Geometry check sheet. Reference: the model listing, model coordinates, mm. A direction names the side the tool comes from. Give positions to 0.01 mm unless a question says otherwise; leave off trailing zeros. Order: outer loops, then holes, each group sorted by start corner. A loop starts at its lowest first (then second) coordinate and runs counter-clockwise, first axis right, second up. Notation, with made-up numbers: M 33,59 L 58,59 A30 cw 58,83 Z; hole C -28.5,-15 d9. An arc over 180 degrees is marked long. One line per question, with ' | ' between items. Start each with the question number.
Autodesk Inventor part; units mm, degrees
ref_plane "YZ Plane" through (0, 0, 0) normal (1, 0, 0) x (0, 1, 0)
ref_plane "XZ Plane" through (0, 0, 0) normal (0, 1, 0) x (-1, 0, 0)
ref_plane "XY Plane" through (0, 0, 0) normal (0, 0, 1) x (1, 0, 0)
sketch "Sketch1" plane through (0, 0, 0) normal (0, 1, 0) x (-1, 0, 0)
  line L0 (0, 0) -> (0, -25.4)
  line L1 (0, -25.4) -> (3.175, -25.4)
  line L2 (3.175, -25.4) -> (3.175, -3.175)
  line L3 (3.175, -3.175) -> (25.4, -3.175)
  line L4 (25.4, -3.175) -> (25.4, 0)
  line L5 (25.4, 0) -> (0, 0)
  dimension "d0" = 3.175
  dimension "d1" = 3.175
  dimension "d2" = 25.4
  dimension "d3" = 25.4
extrude "Extrusion1" add sketch "Sketch1" along normal blind 177.8
sketch "Sketch2" plane through (-25.4, 0, 0) normal (0, 0, 1) x (1, 0, 0)
  line L0 (0, 177.8) -> (25.4, 177.8)
  line L1 (0, 0) -> (25.4, 0)
  line L2 (0, 0) -> (0, 177.8)
  point P0 (12.7, 165.1)
  point P1 (12.7, 12.7)
  dimension "d6" = 12.7
  dimension "d7" = 12.7
  dimension "d8" = 12.7
  dimension "d9" = 12.7
hole "Hole1" at (-12.7, 165.1, 0) at (-12.7, 12.7, 0) direction (0, 0, -1) diameter 6.7469 end through all
properties part number "15102898-16-P-0312"
Item 1: Cross-section at A-A, the plane x = -12.7. Record the cut outline in (y, z) (3 decimals), plus the area to 3 significant figures.
Item 2: Cross-section at D-D, the plane z = -9.5. Record the cut outline in (x, y) (3 decimals), plus the area to 3 significant figures.
Item 3: Depth check by flat-ended pin: pin 1 (11 mm diameter, centred on x = -11, y = 80.5, fed in from -Z) (3 decimals); pin 2 (5.5 mm diameter, centred on x = -12.7, y = 165.1, fed in from +Z). Enter the tip coordinate at first touch or a pass-through.
Item 4: Material ranges on line 1 along Y through (x, z) = (-12.7, -1.45); line 2 along X through (y, z) = (165.1, -2.1); line 3 along X through (y, z) = (132, -10) (3 decimals), recorded low to high.
Item 5: Set-up check for faces 1 (the flat face through (-14, 88, -3.175)), 2 (the flat face through (0, 88, -13)): record each of +Z, -Z, +X, -X, +Y, -Y from which the full face is reachable in a straight line by a thin tool's end or side.
Item 6: Cross-section at B-B, the plane y = 165.1. Record the cut outline in (x, z) (3 decimals).
Item 7: Mould release check, pull along Y, two halves, no side actions. Record for faces 3 (the flat face through (-2, 177.8, -7)), 4 (the flat face through (-25.4, 88, -2)), 5 (the cylindrical face through (-12.85, 168.47, -1.61)), 6 (the flat face through (-2, 0, -7)): released by +Y, released by -Y, zero draft, split by the parting line, or undercut.
Item 8: Cross-section at C-C, the plane y = 65. Record the cut outline in (x, z) (3 decimals).
Outcome:
1) outline: M 0,-3.175 L 9.327,-3.175 L 9.327,0 L 0,0 Z; M 16.073,-3.175 L 161.727,-3.175 L 161.727,0 L 16.073,0 Z; M 168.473,-3.175 L 177.8,-3.175 L 177.8,0 L 168.473,0 Z | area: 522 mm²
2) outline: M -3.175,0 L 0,0 L 0,177.8 L -3.175,177.8 Z | area: 565 mm²
3) pin 1: stops at z = -3.175 | pin 2: passes through
4) line 1: y = 0 to 9.33, 16.07 to 161.73, 168.47 to 177.8 | line 2: x = -25.4 to -16.07, -9.33 to 0 | line 3: x = -3.175 to 0
5) face 1: -Z, -X, +Y, -Y | face 2: +Z, -Z, +X, +Y, -Y
6) outline: M -25.4,-3.175 L -16.073,-3.175 L -16.073,0 L -25.4,0 Z; M -9.327,-3.175 L -3.175,-3.175 L -3.175,-25.4 L 0,-25.4 L 0,0 L -9.327,0 Z
7) face 3: released by +Y | face 4: zero draft | face 5: undercut | face 6: released by -Y
8) outline: M -25.4,-3.175 L -3.175,-3.175 L -3.175,-25.4 L 0,-25.4 L 0,0 L -25.4,0 Z
